Part model, mm, in its own coordinate system. A direction names the side the tool comes from. Round coordinates to 2 decimals unless told otherwise and drop trailing zeros. Order: outer loops, then holes, each group sorted by start corner. A loop starts at its lowest first (then second) coordinate and runs counter-clockwise, first axis right, second up. Notation, with made-up numbers: (-29, 48.5) - (-15, 48.5) arc R23 cw to (-15, 69.5) - close; hole circle Ø6 at (80, -23.5). An arc over 180 degrees is marked (long way). Answer as a JSON object with one key per item and string values.
Autodesk Inventor part; units mm, degrees
ref_plane "YZ Plane" through (0, 0, 0) normal (1, 0, 0) x (0, 1, 0)
ref_plane "XZ Plane" through (0, 0, 0) normal (0, 1, 0) x (-1, 0, 0)
ref_plane "XY Plane" through (0, 0, 0) normal (0, 0, 1) x (1, 0, 0)
sketch "Sketch1" plane through (0, 0, 0) normal (0, 1, 0) x (-1, 0, 0)
  line L0 (0, 0) -> (46, 0)
  line L1 (46, 0) -> (46, -60)
  line L2 (46, -60) -> (0, -60)
  line L3 (0, -60) -> (0, 0)
  dimension "d0" = 46
  dimension "d1" = 60
extrude "Extrusion1" add sketch "Sketch1" along normal blind 3
sketch "Sketch2" plane through (0, 0, 0) normal (0, -1, 0) x (1, 0, 0)
  line L0 (-46, -60) -> (-46, 0)
  line L1 (-46, 0) -> (0, 0)
  line L2 (-46, -60) -> (-43, -60)
  line L3 (-43, -60) -> (-43, 0)
  line L4 (-43, 0) -> (-46, 0)
  line L5 (-46, 0) -> (-46, -60)
  line L6 (0, -60) -> (-46, -60)
  line L7 (0, -60) -> (-3, -60)
  line L8 (-3, -60) -> (-3, 0)
  line L9 (-3, 0) -> (0, 0)
  line L10 (0, 0) -> (0, -60)
  dimension "d4" = 3
  dimension "d5" = 3
  dimension "d6" = 60
extrude "Extrusion2" add sketch "Sketch2" along normal blind 31 contours L0 L1 L3 L2 | L8 L1 L10 L6
sketch "Sketch3" plane through (0, 3, 0) normal (1, 0, 0) x (0, 0, -1)
  line L0 (0, -3) -> (0, -34)
  line L1 (60, -3) -> (60, -34)
  line L2 (60, -18.5) -> (48.5, -18.5)
  circle A0 centre (40.5, -18.5) radius 1
  circle A1 centre (48.5, -26.5) radius 1
  circle A2 centre (56.5, -18.5) radius 1
  circle A3 centre (48.5, -10.5) radius 1
  line L3 (60, -34) -> (0, -34)
  dimension "d16" = 11.5
  dimension "d17" = 2
  dimension "d18" = 8
  dimension "d21" = 360
  dimension "d40" = 15.5
extrude "Extrusion3" cut sketch "Sketch3" against normal blind 3
sketch "Sketch4" plane through (0, 3, 0) normal (1, 0, 0) x (0, 0, -1)
  point P0 (0, -3)
sketch "Sketch5" plane through (0, 3, 0) normal (1, 0, 0) x (0, 0, -1)
  line L0 (0, -34) -> (0, 0)
  line L1 (0, -26) -> (8, -34)
  line L2 (60, -34) -> (0, -34)
  line L3 (52, -34) -> (60, -26)
  line L4 (60, 0) -> (60, -34)
  point P0 (0, -3)
  dimension "d25" = 8
  dimension "d26" = 8
  dimension "d27" = 8
  dimension "d28" = 8
extrude "Extrusion4" cut sketch "Sketch5" against normal blind 50
sketch "Sketch6" plane through (0, 3, 0) normal (0, 1, 0) x (1, 0, 0)
  line L0 (-3, 60) -> (-3, 0)
  line L1 (-43, 60) -> (-3, 60)
  line L2 (-3, 60) -> (-3, 50)
  line L3 (-3, 50) -> (-43, 50)
  line L4 (-43, 50) -> (-43, 60)
  line L5 (-43, 0) -> (-3, 0)
  line L6 (-3, 0) -> (-43, 0)
  line L7 (-43, 0) -> (-43, 10)
  line L8 (-43, 10) -> (-3, 10)
  line L9 (-3, 10) -> (-3, 0)
  point P0 (0, 0)
  dimension "d31" = 10
  dimension "d32" = 40
  dimension "d33" = 10
extrude "Extrusion5" cut sketch "Sketch6" against normal blind 10
sketch "Sketch8" plane through (-46, 3, -60) normal (-1, 0, 0) x (0, 0, 1)
  line L0 (8, -34) -> (52, -34)
  line L1 (11.5, -34) -> (11.5, -18.5)
  line L2 (11.5, -34) -> (27, -34) construction
  circle A0 centre (11.5, -18.5) radius 1.5
  line L3 (0, -26) -> (0, 0)
  point P0 (60, -3)
  dimension "d38" = 15.5
  dimension "d39" = 90
  dimension "d41" = 3
  dimension "d42" = 11.5
extrude "Extrusion7" cut sketch "Sketch8" against normal blind 3
sketch "Sketch9" plane through (0, 3, 0) normal (1, 0, 0) x (0, 0, -1)
  line L0 (0, -26) -> (0, 0)
  line L1 (0, -18.5) -> (11.5, -18.5)
  line L2 (0, -18.5) -> (11.5, -18.5) construction
  line L3 (52, -34) -> (8, -34)
  circle A0 centre (11.5, -10.5) radius 1
  circle A1 centre (11.5, -26.5) radius 1
  point P0 (0, -3)
  dimension "d47" = 11.5
  dimension "d49" = 15.5
  dimension "d50" = 2
  dimension "d51" = 8
extrude "Extrusion8" cut sketch "Sketch9" against normal blind 50
sketch "Sketch10" plane through (-46, 3, -60) normal (-1, 0, 0) x (0, 0, 1)
  line L0 (10, 0) -> (10, -3)
  line L1 (10, 0) -> (0, -10)
  line L2 (0, 0) -> (0, -26)
  line L3 (0, 0) -> (60, 0)
  line L4 (50, 0) -> (60, -10)
  line L5 (60, -26) -> (60, 0)
  point P0 (60, -3)
  dimension "d54" = 10
  dimension "d55" = 10
  dimension "d56" = 10
  dimension "d57" = 10
extrude "Extrusion9" cut sketch "Sketch10" against normal blind 50
properties part number "second_junction"
Item 1: Cut at C-C (z = -24.5). Write the cut outline in (x, y), plus the area to 3 significant figures.
Taken from the geometry:
{"outline": "(-46, -31) - (-43, -31) - (-43, 0) - (-3, 0) - (-3, -31) - (0, -31) - (0, 3) - (-46, 3) - close", "area": "324 mm2"}
Item 2: Two-plate mould, pull along Y, no slides. Class faces 4 (the flat face through (0, -14, -30)), 5 (the flat face through (-45, -31, -30)), 6 (the cylindrical face through (-1.5, -16.1, -55.7)): pulls with the +Y half, pulls with the -Y half, needs draft (parallel to the pull), parting line crosses it, or undercut.
Taken from the geometry:
{"face 4": "needs draft", "face 5": "pulls with the -Y half", "face 6": "undercut"}
Item 3: Cut at D-D (y = -21). Write the cut outline in (x, z), plus the area to 3 significant figures.
Taken from the geometry:
{"outline": "(-46, -60) - (-43, -60) - (-43, 0) - (-46, 0) - close; (-3, -60) - (0, -60) - (0, 0) - (-3, 0) - close", "area": "360 mm2"}
Item 4: Probe L1, parallel to Y at x = -44.4, z = -11.5; L2, parallel to X at y = -12, z = -20; L3, parallel to Z at x = -1, y = -7. List the from-to ranges inside material, lowest first. Write a range as from..to.
Taken from the geometry:
{"L1": "-31..-24.5, -22.5..-8.5, -6.5..3", "L2": "-46..-43, -3..0", "L3": "-60..-49.37, -47.63..-12.37, -10.63..0"}
Item 5: Cut at A-A (y = -2). Write the cut outline in (x, z).
Taken from the geometry:
{"outline": "(-46, -55) - (-43, -55) - (-43, -5) - (-46, -5) - close; (-3, -55) - (0, -55) - (0, -5) - (-3, -5) - close"}
Item 6: Tool access for faces 1 (the flat face through (-23, 0, -30)), 2 (the flat face through (-23, 2, -10)), 3 (the cylindrical face through (-1.479, -7.2, -49.454)): list every direction of +Z, -Z, +X, -X, +Y, -Y with a clear straight run to the whole face (end or side of a thin tool).
Taken from the geometry:
{"face 1": "+Z, -Z, -Y", "face 2": "+Z, +Y, -Y", "face 3": "+X"}
Item 7: Drop flat-ended pins along their axis: P1, Ø3.5, axis at x = -15, y = 2, coming from the +Z side; P2, Ø1.8, axis at y = -15.5, z = -48.5, coming from the -X side; P3, Ø0.9, axis at x = -25.5, y = 1.5, coming from the -Z side. Give the stop position or say it passes through.
Taken from the geometry:
{"P1": "z = -10", "P2": "x = -3", "P3": "z = -50"}
Item 8: Cut at B-B (z = -11.5). Write the cut outline in (x, y), plus the area to 3 significant figures.
Taken from the geometry:
{"outline": "(-46, -31) - (-43, -31) - (-43, -24.5) - (-46, -24.5) - close; (-46, -22.5) - (-43, -22.5) - (-43, -8.5) - (-46, -8.5) - close; (-46, -6.5) - (-43, -6.5) - (-43, 0) - (-3, 0) - (-3, -6.5) - (0, -6.5) - (0, 3) - (-46, 3) - close; (-3, -31) - (0, -31) - (0, -24.5) - (-3, -24.5) - close; (-3, -22.5) - (0, -22.5) - (0, -8.5) - (-3, -8.5) - close", "area": "300 mm2"}
